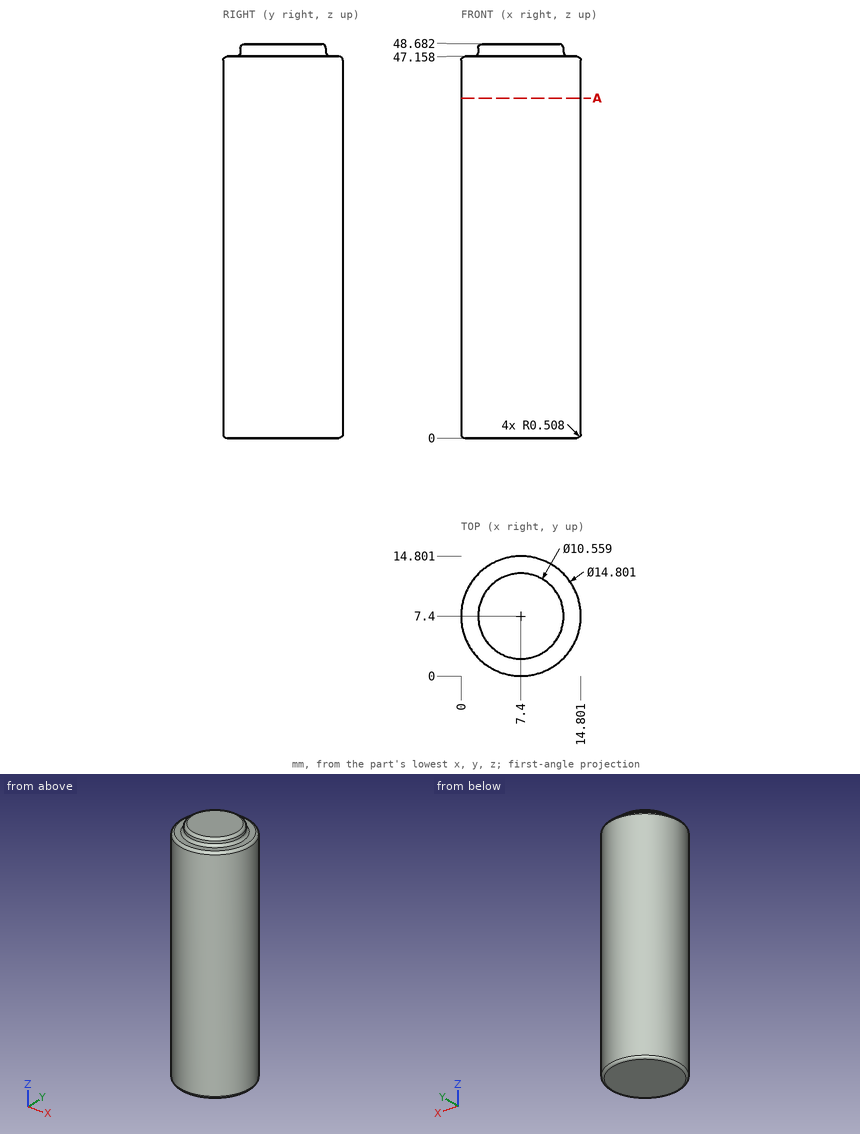
Job drawing, mm, ordinate dimensions from the low corner. One solid piece. Round coordinates to 2 decimals unless told otherwise and drop trailing zeros. Order: outer loops, then holes, each group sorted by start corner. A loop starts at its lowest first (then second) coordinate and runs counter-clockwise, first axis right, second up. Notation, with made-up numbers: (67, -25.75) -> (116, -25.75) arc R27 ccw to (116, 13.25) -> close; hole circle Ø10 at (21, -30.75). An arc over 180 degrees is marked (long way). Answer in a Markdown table with one row per item.
1) Band-saw the part on A-A on z = 42. Give the cut face in (x, y), and give its area (3 significant figures).
Values:
| item | result |
|---|---|
| outline | circle Ø14.8 at (7.4, 7.4) |
| area | 172 mm2 |
2) Pin check, flat tips, straight feed: P1, Ø2, axis at y = 11, z = 40, coming from the -X side; P2, Ø5, axis at x = 3, z = 8.5, coming from the +Y side; P3, Ø3, axis at y = 4.5, z = 16.5, coming from the +X side. Stop position of each tip, or through.
Values:
| item | result |
|---|---|
| P1 | x = 0.47 |
| P2 | y = 14.55 |
| P3 | x = 14.67 |
3) Wall check: L1, parallel to Z at x = 1.25, y = 5.25; L2, parallel to X at y = 7.75, z = 42.5; L3, parallel to Y at x = 1.75, z = 11. Give the ranges that are in metal, low to high.
Values:
| item | result |
|---|---|
| L1 | 0 to 47.16 |
| L2 | 0.01 to 14.79 |
| L3 | 2.62 to 12.18 |
